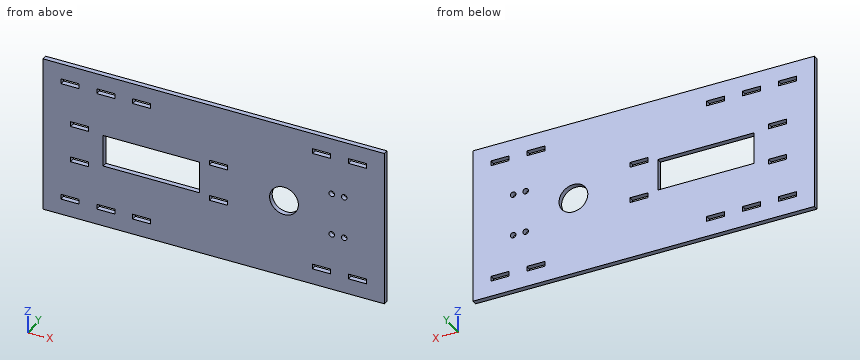
```python
from build123d import *

# Parameters (mm, degrees)
SKETCH1_W               = 215.9
SKETCH1_H               = 100
BOSS_EXTRUDE1_DEPTH     = 3.175
SKETCH3_W               = 11.35
SKETCH3_H               = 3.175
CUT_EXTRUDE2_DEPTH      = 3.175
SKETCH4_W               = 11.35
SKETCH4_H               = 3.175
CUT_EXTRUDE3_DEPTH      = 3.175
SKETCH5_W               = 60.96
SKETCH5_H               = 20.32
CUT_EXTRUDE4_DEPTH      = 1
CUT_EXTRUDE4_DEPTH_BACK = 3.175
SKETCH7_R               = 9.1
CUT_EXTRUDE6_DEPTH      = 3.175
SKETCH8_R               = 1.778
CUT_EXTRUDE7_DEPTH      = 3.175
SKETCH9_W               = 11.35
SKETCH9_H               = 3.175
CUT_EXTRUDE8_DEPTH      = 3.175


with BuildPart() as part:
    # Sketch1 → Boss-Extrude1 (new body)
    with BuildSketch(Plane(origin=(0, 0, 0), x_dir=(1, 0, 0), z_dir=(0, 1, 0))):
        with Locations((-1.255776173, 17.463898917)):
            Rectangle(SKETCH1_W, SKETCH1_H)
    extrude(amount=BOSS_EXTRUDE1_DEPTH)

    # Sketch3 → Cut-Extrude2 (cut)
    with BuildSketch(Plane(origin=(0, 3.175, 0), x_dir=(1, 0, 0), z_dir=(0, 1, 0))):
        with Locations((-92.180776173, 55.876398917)):
            Rectangle(SKETCH3_W, SKETCH3_H)
        with Locations((-46.780776173, 55.876398917)):
            Rectangle(SKETCH3_W, SKETCH3_H)
        with Locations((-69.480776173, 55.876398917)):
            Rectangle(SKETCH3_W, SKETCH3_H)
        with Locations((66.969233827, 55.876398917)):
            Rectangle(SKETCH3_W, SKETCH3_H)
        with Locations((89.669223827, 55.876398917)):
            Rectangle(SKETCH3_W, SKETCH3_H)
    extrude(amount=-CUT_EXTRUDE2_DEPTH, mode=Mode.SUBTRACT)

    # Sketch4 → Cut-Extrude3 (cut)
    with BuildSketch(Plane(origin=(0, 3.175, 0), x_dir=(1, 0, 0), z_dir=(0, 1, 0))):
        with Locations((-92.180776173, -20.948601083)):
            Rectangle(SKETCH4_W, SKETCH4_H)
        with Locations((-69.480776173, -20.948601083)):
            Rectangle(SKETCH4_W, SKETCH4_H)
        with Locations((-46.780776173, -20.948601083)):
            Rectangle(SKETCH4_W, SKETCH4_H)
        with Locations((66.969233827, -20.948601083)):
            Rectangle(SKETCH4_W, SKETCH4_H)
        with Locations((89.669223827, -20.948601083)):
            Rectangle(SKETCH4_W, SKETCH4_H)
    extrude(amount=-CUT_EXTRUDE3_DEPTH, mode=Mode.SUBTRACT)

    # Sketch5 → Cut-Extrude4 (cut, two sides)
    with BuildSketch(Plane(origin=(0, 3.175, 0), x_dir=(1, 0, 0), z_dir=(0, 1, 0))) as cut_extrude4_sk:
        with Locations((-40.625776173, 17.503898917)):
            Rectangle(SKETCH5_W, SKETCH5_H)
    extrude(amount=CUT_EXTRUDE4_DEPTH, mode=Mode.SUBTRACT)
    extrude(cut_extrude4_sk.sketch, amount=-CUT_EXTRUDE4_DEPTH_BACK, mode=Mode.SUBTRACT)

    # Sketch7 → Cut-Extrude6 (cut)
    with BuildSketch(Plane(origin=(0, 3.175, 0), x_dir=(1, 0, 0), z_dir=(0, 1, 0))):
        with Locations((43.194223827, 17.463898917)):
            Circle(SKETCH7_R)
    extrude(amount=-CUT_EXTRUDE6_DEPTH, mode=Mode.SUBTRACT)

    # Sketch8 → Cut-Extrude7 (cut)
    with BuildSketch(Plane(origin=(0, 3.175, 0), x_dir=(1, 0, 0), z_dir=(0, 1, 0))):
        with Locations((73.394823827, 30.938498917)):
            Circle(SKETCH8_R)
        with Locations((81.294223827, 3.989098917)):
            Circle(SKETCH8_R)
        with Locations((73.394823827, 3.989098917)):
            Circle(SKETCH8_R)
        with Locations((81.294223827, 30.938498917)):
            Circle(SKETCH8_R)
    extrude(amount=-CUT_EXTRUDE7_DEPTH, mode=Mode.SUBTRACT)

    # Sketch9 → Cut-Extrude8 (cut)
    with BuildSketch(Plane(origin=(0, 3.175, 0), x_dir=(1, 0, 0), z_dir=(0, 1, 0))):
        with Locations((-86.004776173, 5.756398917)):
            Rectangle(SKETCH9_W, SKETCH9_H)
        with Locations((-86.004776173, 29.251398917)):
            Rectangle(SKETCH9_W, SKETCH9_H)
        with Locations((1.705223827, 5.756398917)):
            Rectangle(SKETCH9_W, SKETCH9_H)
        with Locations((1.705223827, 29.251398917)):
            Rectangle(SKETCH9_W, SKETCH9_H)
    extrude(amount=-CUT_EXTRUDE8_DEPTH, mode=Mode.SUBTRACT)


solid = part.part
```
Check sheet for the modelled part. Datum: model origin and axes. Units: mm. Coordinates: 2 decimals unless noted, no trailing zeros. Write each loop counter-clockwise with the first axis right and the second up, starting at its lowest first coordinate (ties: lowest second). Pieces come first, ordered by that corner, then holes. Notation, with made-up numbers: (49.5, -33.5) - (65.5, -33.5) arc R12 ccw to (65.5, -13.5) - close; hole circle Ø3 at (-29, 3). An arc over 180 degrees is marked (long way). One line per question, with ' | ' between items.
Item 1: Sectioned sample at D-D on x = -45.5. Record the boundary of the cut face in (y, z) (3 decimals), plus the area to 3 significant figures.
Determined:
outline: (0, -67.464) - (3.175, -67.464) - (3.175, -57.464) - (0, -57.464) - close; (0, -54.289) - (3.175, -54.289) - (3.175, -27.664) - (0, -27.664) - close; (0, -7.344) - (3.175, -7.344) - (3.175, 19.361) - (0, 19.361) - close; (0, 22.536) - (3.175, 22.536) - (3.175, 32.536) - (0, 32.536) - close | area: 233 mm2
Item 2: Gauge pin test, flat end, axial feed: P1, Ø12, axis at x = 75, z = 17, coming from the -Y side. Record the tip position at first contact, or that the pin passes through.
Determined:
P1: stops at y = 0
Item 3: Sectioned sample at A-A on x = 67. Record the boundary of the cut face in (y, z) (3 decimals), plus the area to 3 significant figures.
Determined:
outline: (0, -67.464) - (3.175, -67.464) - (3.175, -57.464) - (0, -57.464) - close; (0, -54.289) - (3.175, -54.289) - (3.175, 19.361) - (0, 19.361) - close; (0, 22.536) - (3.175, 22.536) - (3.175, 32.536) - (0, 32.536) - close | area: 297 mm2
Item 4: Sectioned sample at B-B on z = -23. Record the boundary of the cut face in (x, y) (3 decimals), plus the area to 3 significant figures.
Determined:
outline: (-109.206, 0) - (-71.106, 0) - (-71.106, 3.175) - (-109.206, 3.175) - close; (-10.146, 0) - (35.972, 0) - (35.972, 3.175) - (-10.146, 3.175) - close; (50.417, 0) - (106.694, 0) - (106.694, 3.175) - (50.417, 3.175) - close | area: 446 mm2
Item 5: Thickness scan on line 1 (Z direction, x = -91.5, y = 1); line 2 (Z direction, x = 91.5, y = 1.55); line 3 (Z direction, x = -51.5, y = 2.25). Record the ranges inside material, lowest first. Write a range as [from, to].
Determined:
line 1: z = [-67.46, -57.46], [-54.29, -30.84], [-27.66, -7.34], [-4.17, 19.36], [22.54, 32.54] | line 2: z = [-67.46, -57.46], [-54.29, 19.36], [22.54, 32.54] | line 3: z = [-67.46, -57.46], [-54.29, -27.66], [-7.34, 19.36], [22.54, 32.54]
Item 6: Sectioned sample at C-C on x = 42. Record the boundary of the cut face in (y, z) (3 decimals).
Determined:
outline: (0, -67.464) - (3.175, -67.464) - (3.175, -26.485) - (0, -26.485) - close; (0, -8.443) - (3.175, -8.443) - (3.175, 32.536) - (0, 32.536) - close
